```python
from build123d import *

# Parameters (mm, degrees)
SKETCH1_W                       = 5
SKETCH1_H                       = 20
SKETCH1_W_2                     = 14
SKETCH1_H_2                     = 3
BOSS_EXTRUDE1_DEPTH             = 30
SKETCH4_W                       = 4
SKETCH4_H                       = 2
SKETCH4_W_2                     = 2
SKETCH4_H_2                     = 8
BOSS_EXTRUDE2_DEPTH             = 60
SKETCH4_4_W                     = 2
SKETCH4_4_H                     = 20
BOSS_EXTRUDE3_DEPTH             = 20
SKETCH4_5_W                     = 2
SKETCH4_5_H                     = 8
SKETCH4_5_H_2                   = 20
CUT_EXTRUDE1_DEPTH              = 10
SKETCH2_R                       = 5
SKETCH2_R_2                     = 2.5
BOSS_EXTRUDE4_DEPTH             = 30
BOSS_EXTRUDE4_DIRECTION_2_REACH = 76.54
FILLET1_R                       = 5


with BuildPart() as part:
    # Sketch1 → Boss-Extrude1 (new body)
    with BuildSketch(Plane(origin=(0, 0, 0), x_dir=(0, 0, -1), z_dir=(1, 0, 0))):
        with Locations((0, 11.5)):
            Rectangle(SKETCH1_W, SKETCH1_H)
        Rectangle(SKETCH1_W_2, SKETCH1_H_2)
    extrude(amount=BOSS_EXTRUDE1_DEPTH)



with BuildPart() as body_2:
    # Sketch4 → Boss-Extrude2 (new body)
    with BuildSketch(Plane(origin=(0, 0, 0), x_dir=(1, 0, 0), z_dir=(0, 1, 0))):
        with Locations((18, 31.5)):
            Rectangle(SKETCH4_W, SKETCH4_H)
        with Locations((15, 31.5)):
            Rectangle(SKETCH4_W_2, SKETCH4_H)
        with Locations((12, 31.5)):
            Rectangle(SKETCH4_W, SKETCH4_H)
        with Locations((15, 26.5)):
            Rectangle(SKETCH4_W_2, SKETCH4_H_2)
    extrude(amount=BOSS_EXTRUDE2_DEPTH)


with BuildPart() as part_1:
    add(part.part)

    add(body_2.part)  # Boss-Extrude3 merges body 2
    # Sketch4<4> → Boss-Extrude3 (add)
    with BuildSketch(Plane(origin=(0, 0, 0), x_dir=(1, 0, 0), z_dir=(0, 1, 0))):
        with Locations((15, 12.5)):
            Rectangle(SKETCH4_4_W, SKETCH4_4_H)
    extrude(amount=BOSS_EXTRUDE3_DEPTH)

    # Sketch4<5> → Cut-Extrude1 (cut)
    with BuildSketch(Plane(origin=(0, 0, 0), x_dir=(1, 0, 0), z_dir=(0, 1, 0))):
        with Locations((15, 26.5)):
            Rectangle(SKETCH4_5_W, SKETCH4_5_H)
        with Locations((15, 12.5)):
            Rectangle(SKETCH4_5_W, SKETCH4_5_H_2)
    extrude(amount=CUT_EXTRUDE1_DEPTH, mode=Mode.SUBTRACT)

    # Sketch2 → Boss-Extrude4 (add)
    with BuildSketch(Plane.XY):
        with Locations((15, 55)):
            Circle(SKETCH2_R)
        with Locations((15, 55)):
            Circle(SKETCH2_R_2, mode=Mode.SUBTRACT)
    extrude(amount=BOSS_EXTRUDE4_DEPTH)

    # Boss-Extrude4 direction 2: up to this face of the body (flat: up to its plane)
    boss_extrude4_direction_2_end = Plane(part_1.part.faces().sort_by_distance((15, 30, -32.5))[0])
    # Sketch2 → Boss-Extrude4 direction 2 (add, up to the picked face)
    with BuildSketch(Plane.XY, mode=Mode.PRIVATE) as boss_extrude4_direction_2_sk1:
        with Locations((15, 55)):
            Circle(SKETCH2_R)
        with Locations((15, 55)):
            Circle(SKETCH2_R_2, mode=Mode.SUBTRACT)
    boss_extrude4_direction_2_tool1 = split(extrude(boss_extrude4_direction_2_sk1.sketch, amount=-BOSS_EXTRUDE4_DIRECTION_2_REACH, mode=Mode.PRIVATE), bisect_by=boss_extrude4_direction_2_end, keep=Keep.BOTH, mode=Mode.PRIVATE)
    add(boss_extrude4_direction_2_tool1.solids().sort_by(Axis((10.141421, 55, 0), (0, 0, -1)))[0])

    # Fillet1
    fillet1_edges = [part_1.edges().sort_by_distance(p)[0] for p in [
        (15, 20, -22.5),
        (15, 10, -30.5),
    ]]
    fillet(fillet1_edges, radius=FILLET1_R)


solid = part_1.part
```
Can you work these out from the model? Positions are in its coordinate system, mm. A direction names the side the tool comes from. Round coordinates to 2 decimals unless told otherwise and drop trailing zeros. Order: outer loops, then holes, each group sorted by start corner. A loop starts at its lowest first (then second) coordinate and runs counter-clockwise, first axis right, second up. Notation, with made-up numbers: (54, 74.25) -> (80, 74.25) arc R18 ccw to (80, 105.25) -> close; hole circle Ø8 at (65.25, 38.25). An arc over 180 degrees is marked (long way). Return JSON: item names as keys, results as strings. Group by question number.
1. If we section it at C-C, the plane y = 14: Write out the boundary of the cut face in (x, z).
2. Which directions (+Z, -Z, +X, -X, +Y, -Y) give clear straight access to the entire face, cutting with the end or side of a thin tool? Please do faces 1 (the face through (23, 1.5, -5)), 2 (the face through (11, 59, -30.5)), 3 (the face through (13.8, 27.1, -30.5)), 4 (the face through (15, 0, -32)), 5 (the face through (15, 11, 2.5)).
3. If we section it at A-A, the plane z = 1: Write out the boundary of the cut face in (x, y), then the cut area to 3 significant figures.
4. If we section it at B-B, the plane x = 2.5: Write out the boundary of the cut face in (y, z).
5. If we section it at D-D, the plane x = 11.75: Write out the boundary of the cut face in (y, z), then the cut area to 3 significant figures.
6. Will these pins go through, and if not, where does the flat tip stop? pin 1 (6 mm diameter, centred on y = 50, z = 3, fed in from +X); pin 2 (1 mm diameter, centred on x = 26, y = 17, fed in from -Z); pin 3 (14 mm diameter, centred on y = 16.5, z = -19, fed in from +X); pin 4 (1.5 mm diameter, centred on y = 48, z = 4, fed in from -X) (3 decimals).
7. We'd pull the mould along Z, two halves only. Please class faces 6 (the face through (15, 21.5, 0)), 7 (the face through (15, 37, -22.5)), 8 (the face through (15, 20, -10)): released by +Z, released by -Z, zero draft, split by the parting line, or undercut.
8. I need wall thicknesses on line 1 (Y direction, x = 15, z = -8); line 2 (Z direction, x = 12.75, y = 18); line 3 (X direction, y = 55, z = -7.5). Which ranges of each line are inside material? Lowest first, please. Write a range as [from, to].
Output values:
{
 "1": {"outline": "(0, -2.5) -> (14, -2.5) -> (14, -30.5) -> (10, -30.5) -> (10, -32.5) -> (20, -32.5) -> (20, -30.5) -> (16, -30.5) -> (16, -2.5) -> (30, -2.5) -> (30, 2.5) -> (0, 2.5) -> close"},
 "2": {"face 1": "+X, -X", "face 2": "+Z, -X, +Y", "face 3": "-Y", "face 4": "-Z, +X, -X, -Y", "face 5": "+Z, +X, -X"},
 "3": {"outline": "(0, -1.5) -> (30, -1.5) -> (30, 21.5) -> (0, 21.5) -> close; circle Ø10 at (15, 55); hole circle Ø5 at (15, 55)", "area": "749 mm²"},
 "4": {"outline": "(-1.5, -7) -> (1.5, -7) -> (1.5, -2.5) -> (21.5, -2.5) -> (21.5, 2.5) -> (1.5, 2.5) -> (1.5, 7) -> (-1.5, 7) -> close"},
 "5": {"outline": "(-1.5, -7) -> (1.5, -7) -> (1.5, -2.5) -> (21.5, -2.5) -> (21.5, 2.5) -> (1.5, 2.5) -> (1.5, 7) -> (-1.5, 7) -> close; (0, -32.5) -> (60, -32.5) -> (60, -30.5) -> (58.8, -30.5) -> (58.8, 30) -> (51.2, 30) -> (51.2, -30.5) -> (0, -30.5) -> close", "area": "722 mm²"},
 "6": {"pin 1": "x = 19.58", "pin 2": "z = -2.5", "pin 3": "x = 16", "pin 4": "through"},
 "7": {"face 6": "zero draft", "face 7": "released by +Z", "face 8": "undercut"},
 "8": {"line 1": "[10, 20], [50, 52.5], [57.5, 60]", "line 2": "[-32.5, -30.5], [-2.5, 2.5]", "line 3": "[10, 12.5], [17.5, 20]"}
}
